Model file for the job. Use its own axes, mm. Face numbers are marked on the shaded views. A direction names the side the tool comes from. Round coordinates to 2 decimals unless told otherwise and drop trailing zeros. Order: outer loops, then holes, each group sorted by start corner. A loop starts at its lowest first (then second) coordinate and runs counter-clockwise, first axis right, second up. Notation, with made-up numbers: (3.5, 52) -> (51.5, 52) arc R25 cw to (51.5, 85) -> close; hole circle Ø6 at (31.5, -27.75). An arc over 180 degrees is marked (long way). Put each result on its own line as item: value. Start each with the question number.
Q1. 3-axis set-ups, long thin cutter, end or side, ignore diameter. For the marked faces 4, 5, 6 and 7: which of +Z, -Z, +X, -X, +Y, -Y reach the whole face in a straight line?
Q2. Cut at D-D, the plane x = 0. List the corners of the cut face in (y, z).
Q3. Cut at A-A, the plane x = -20. List the corners of the cut face in (y, z), and give its area (3 significant figures).
Q4. Cut at C-C, the plane z = 2.25. List the corners of the cut face in (x, y), and give its area (3 significant figures).
Q5. Probe L1, parallel to Z at x = 6.5, y = -0.5; L2, parallel to Y at x = -20, z = 16.55; L3, parallel to X at y = 0.5, z = 10.75. List the from-to ranges inside material, lowest first.
Q6. Flat gauge pins, fed straight in: P1, Ø1.8, axis at y = 1.5, z = 20, coming from the -X side; P2, Ø0.8, axis at x = 6.5, y = 1, coming from the +Z side; P3, Ø1.6, axis at x = 9, y = 0, coming from the +Z side; P4, Ø3, axis at x = 7.5, y = 3, coming from the -Z side. Where does each tip first touch, or does it go through?
Q7. Cut at B-B, the plane y = 0. List the corners of the cut face in (x, z).
Q8. Pull direction Z, two halves, no side cores. Call the marked faces 1, 2 and 3: released by +Z, released by -Z, zero draft, split by the parting line, or undercut.
from build123d import *

# Parameters (mm, degrees)
SKETCH_W     = 23
SKETCH_H     = 12
PAD_DEPTH    = 23
SKETCH001_W  = 12
SKETCH001_H  = 2
PAD001_DEPTH = 5.5
SKETCH002_W  = 12
SKETCH002_H  = 2
PAD002_DEPTH = 5.5
SKETCH003_R  = 1
POCKET_DEPTH = 5
SKETCH004_R  = 3
PAD003_DEPTH = 3
SKETCH006_W  = 5
SKETCH006_H  = 5
PAD004_DEPTH = 3
FILLET_R     = 2


with BuildPart() as part:
    # Sketch → Pad (new body)
    with BuildSketch(Plane.XY):
        with Locations((-5.5, 0)):
            Rectangle(SKETCH_W, SKETCH_H)
    extrude(amount=PAD_DEPTH)

    # Sketch001 (on Face2 of Pad) → Pad001 (join)
    with BuildSketch(Plane.YZ.offset(6)):
        with Locations((0, 16)):
            Rectangle(SKETCH001_W, SKETCH001_H)
    extrude(amount=PAD001_DEPTH)

    # Sketch002 (on Face2 of Pad001) → Pad002 (join)
    with BuildSketch(Plane(origin=(-17, 0, 0), x_dir=(0, -1, 0), z_dir=(-1, 0, 0))):
        with Locations((0, 16)):
            Rectangle(SKETCH002_W, SKETCH002_H)
    extrude(amount=PAD002_DEPTH)

    # Sketch003 (on Face12 of Pad002) → Pocket (cut)
    with BuildSketch(Plane.XY.offset(17)):
        with Locations((-20, 0)):
            Circle(SKETCH003_R)
        with Locations((9, 0)):
            Circle(SKETCH003_R)
    extrude(amount=-POCKET_DEPTH, mode=Mode.SUBTRACT)

    # Sketch004 (on Face9 of Pocket) → Pad003 (join)
    with BuildSketch(Plane.XY.offset(23)):
        Circle(SKETCH004_R)
    extrude(amount=PAD003_DEPTH)

    # Sketch006 → Pad004 (join)
    with BuildSketch(Plane.YZ.offset(6)):
        with Locations((0, 2.5)):
            Rectangle(SKETCH006_W, SKETCH006_H)
    extrude(amount=PAD004_DEPTH)

    # Fillet
    fillet_edges = [part.edges().sort_by_distance(p)[0] for p in [
        (9, -2.5, 2.5),
        (9, 2.5, 2.5),
        (9, 0, 5),
    ]]
    fillet(fillet_edges, radius=FILLET_R)


solid = part.part
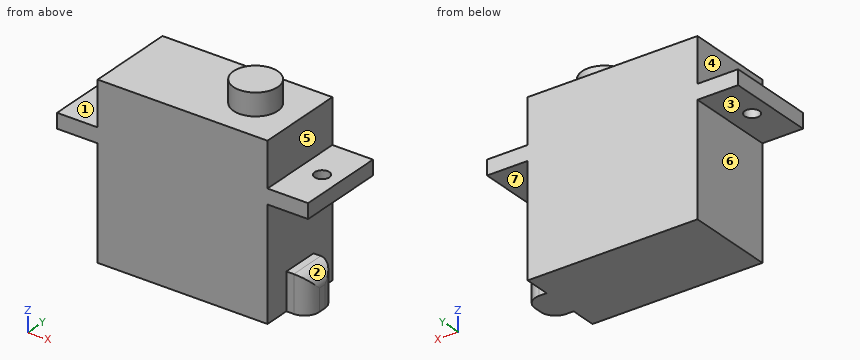
Ans:
1. face 4: +Z, -X, +Y, -Y
1. face 5: +Z, +X, +Y, -Y
1. face 6: -Z, -X, +Y, -Y
1. face 7: +X, +Y, -Y
2. outline: (-6, 0) -> (6, 0) -> (6, 23) -> (3, 23) -> (3, 26) -> (-3, 26) -> (-3, 23) -> (-6, 23) -> close
3. outline: (-6, 15) -> (-1, 15) -> (-1, 17) -> (-6, 17) -> close; (1, 15) -> (6, 15) -> (6, 17) -> (1, 17) -> close
3. area: 20.0 mm^2
4. outline: (-17, -6) -> (6, -6) -> (6, -2.5) -> (7, -2.5) arc R2 ccw to (9, -0.5) -> (9, 0.5) arc R2 ccw to (7, 2.5) -> (6, 2.5) -> (6, 6) -> (-17, 6) -> close
4. area: 289 mm^2
5. L1: z = 0 to 5, 15 to 17
5. L2: y = -6 to -1, 1 to 6
5. L3: x = -17 to 6
6. P1: stops at x = -17
6. P2: stops at z = 17
6. P3: stops at z = 4.6
6. P4: stops at z = 0
7. outline: (-22.5, 15) -> (-21, 15) -> (-21, 17) -> (-22.5, 17) -> close; (-19, 15) -> (-17, 15) -> (-17, 0) -> (9, 0) -> (9, 3) arc R2 ccw to (7, 5) -> (6, 5) -> (6, 15) -> (8, 15) -> (8, 17) -> (6, 17) -> (6, 23) -> (3, 23) -> (3, 26) -> (-3, 26) -> (-3, 23) -> (-17, 23) -> (-17, 17) -> (-19, 17) -> close; (10, 15) -> (11.5, 15) -> (11.5, 17) -> (10, 17) -> close
8. face 1: released by +Z
8. face 2: undercut
8. face 3: released by -Z
